from build123d import *

# Parameters (mm, degrees)
SKETCH021_R     = 10.25
PAD007_DEPTH    = 20
PAD007_FACE1_W  = 40
PAD007_FACE1_H  = 46.7452916506
PAD008_DEPTH    = 4
SKETCH022_R     = 1.75
POCKET007_DEPTH = 6.5
POCKET008_DEPTH = 4
SKETCH024_R     = 2.5
POCKET009_DEPTH = 29.501


with BuildPart() as part:
    # Sketch021 → Pad007 (new body, symmetric)
    with BuildSketch(Plane.XZ):
        with BuildLine():
            Line((23.3726458253, 0), (-23.3726458253, 0))
            Line((-23.3726458253, 0), (-26.8054242847, -7.3616171628))
            ThreePointArc((-26.8054242847, -7.3616171628), (-28, -12.75), (-26.8054242847, -18.1383828372))
            Line((-26.8054242847, -18.1383828372), (-23.3726458253, -25.5))
            Line((-23.3726458253, -25.5), (23.3726458253, -25.5))
            Line((23.3726458253, -25.5), (26.8054242847, -18.1383828372))
            ThreePointArc((26.8054242847, -18.1383828372), (28, -12.75), (26.8054242847, -7.3616171628))
            Line((23.3726458253, 0), (26.8054242847, -7.3616171628))
        make_face()
        with Locations((15.25, -12.75)):
            Circle(SKETCH021_R, mode=Mode.SUBTRACT)
        with Locations((-15.25, -12.75)):
            Circle(SKETCH021_R, mode=Mode.SUBTRACT)
        with BuildLine():
            Line((-7.6671245559, -2.5), (7.6671245559, -2.5))
            ThreePointArc((7.6671245559, -2.5), (2.5, -12.75), (7.6671245559, -23))
            Line((-7.6671245559, -23), (7.6671245559, -23))
            ThreePointArc((-7.6671245559, -23), (-2.5, -12.75), (-7.6671245559, -2.5))
        make_face(mode=Mode.SUBTRACT)
    extrude(amount=PAD007_DEPTH, both=True)

    # Pad007 Face1 → Pad008 (add)
    with BuildSketch(Plane(origin=(0, 0, 0), x_dir=(0, 1, 0), z_dir=(0, 0, 1))):
        Rectangle(PAD007_FACE1_W, PAD007_FACE1_H)
    extrude(amount=PAD008_DEPTH)

    # Sketch022 → Pocket007 (cut)
    with BuildSketch(Plane(origin=(0, 0, 4), x_dir=(-1, 0, 0), z_dir=(0, 0, 1))):
        with Locations((0, 10)):
            Circle(SKETCH022_R)
        with Locations((0, -10)):
            Circle(SKETCH022_R)
    extrude(amount=-POCKET007_DEPTH, mode=Mode.SUBTRACT)

    # Sketch023 (on Face6 of Pocket007) → Pocket008 (cut)
    with BuildSketch(Plane(origin=(0, 0, 4), x_dir=(-1, 0, 0), z_dir=(0, 0, 1))):
        Polygon((2.225, -3.8538130468), (4.45, 0), (2.225, 3.8538130468), (-2.225, 3.8538130468), (-4.45, 0), (-2.225, -3.8538130468), align=None)
    extrude(amount=-POCKET008_DEPTH, mode=Mode.SUBTRACT)

    # Sketch024 (on Face6 of Pocket008) → Pocket009 (cut, through all)
    with BuildSketch(Plane(origin=(0, 0, 4), x_dir=(-1, 0, 0), z_dir=(0, 0, 1))):
        Circle(SKETCH024_R)
    extrude(amount=-POCKET009_DEPTH, mode=Mode.SUBTRACT)


solid = part.part
Input: part model. Units: mm. Frame: model coordinates. A direction names the side the tool comes from. Give positions to 0.01 mm unless a question says otherwise; leave off trailing zeros. Loops run counter-clockwise (first coordinate to the right, second up) from the corner with the lowest first, then second, coordinate; pieces in that order, holes last. Notation, with made-up numbers: (-15.75, 20.5) -> (20.25, 20.5) arc R30 cw to (20.25, 45.5) -> close; hole circle Ø4 at (13.5, 16). An arc over 180 degrees is marked (long way). Answer as a JSON object with one key per item and string values. Group by question number.
Item 1: Pull-direction query (Z, two-part tool) for faces 4 (the flat face through (25.065, -0.28, -3.629)), 5 (the flat face through (-3.322, 1.954, 2.028)), 6 (the cylindrical face through (-2.5, -0.3, -12.9)), 7 (the flat face through (-4, 0, -2.5)); classes: released by +Z, released by -Z, zero draft, split by the parting line, or undercut.
Item 2: Reachability of faces 1 (the cylindrical face through (28, -0.3, -12.8)), 2 (the flat face through (23.373, 0, 2)), 3 (the flat face through (3.353, 1.9, 2.028)) from +Z, -Z, +X, -X, +Y, -Y: full face, straight path, thin tool, end or side. Return the list, or none.
Item 3: Line query: probe 1 along Y at (x, z) = (0, 0.75); probe 2 along Y at (x, z) = (0, -24.45); probe 3 along X at (y, z) = (4, -9.25). Output: solid intervals per line, ascending.
Item 4: Cut plane D-D, the plane z = 2.25. Return the cut outline in (x, y) (3 decimals), and give its area (3 significant figures).
Item 5: Pin query (flat end, axial travel): P1, Ø12, axis at y = -1, z = -22, coming from the +X side; P2, Ø1.2, axis at y = -7.5, z = 1.5, coming from the -X side; P3, Ø4, axis at y = -11, z = -20, coming from the +X side. Return the tip coordinate at first contact, or that it passes through.
Item 6: Cut plane C-C, the plane y = -10. Return the cut outline in (x, z).
Item 7: Cut plane A-A, the plane z = -12.75. Return the cut outline in (x, y).
Item 8: Cut plane B-B, the plane x = 0. Return the cut outline in (y, z), and give its area (3 significant figures).
Checks:
{
 "1": {"face 4": "released by +Z", "face 5": "zero draft", "face 6": "undercut", "face 7": "undercut"},
 "2": {"face 1": "+X, +Y, -Y", "face 2": "+Z, +X, +Y, -Y", "face 3": "+Z"},
 "3": {"probe 1": "y = -20 to -11.75, -8.25 to -3.85, 3.85 to 8.25, 11.75 to 20", "probe 2": "y = -20 to -2.5, 2.5 to 20", "probe 3": "x = -27.51 to -24.88, -5.62 to -2.99, 2.99 to 5.62, 24.88 to 27.51"},
 "4": {"outline": "(-23.373, -20) -> (23.373, -20) -> (23.373, 20) -> (-23.373, 20) -> close; hole (-4.45, 0) -> (-2.225, -3.854) -> (2.225, -3.854) -> (4.45, 0) -> (2.225, 3.854) -> (-2.225, 3.854) -> close; hole circle Ø3.5 at (0, -10); hole circle Ø3.5 at (0, 10)", "area": "1,800 mm²"},
 "5": {"P1": "stops at x = 27.58", "P2": "stops at x = -23.37", "P3": "stops at x = 26.87"},
 "6": {"outline": "(-26.81, -18.14) -> (-23.37, -25.5) -> (23.37, -25.5) -> (26.81, -18.14) arc R12.75 ccw to (26.81, -7.36) -> (23.37, 0) -> (23.37, 4) -> (1.75, 4) -> (1.75, -2.5) -> (7.67, -2.5) arc R12.75 ccw to (7.67, -23) -> (-7.67, -23) arc R12.75 ccw to (-7.67, -2.5) -> (-1.75, -2.5) -> (-1.75, 4) -> (-23.37, 4) -> (-23.37, 0) -> (-26.81, -7.36) arc R12.75 ccw to start; hole circle Ø20.5 at (-15.25, -12.75); hole circle Ø20.5 at (15.25, -12.75)"},
 "7": {"outline": "(-28, -20) -> (-25.5, -20) -> (-25.5, 20) -> (-28, 20) -> close; (-5, -20) -> (-2.5, -20) -> (-2.5, 20) -> (-5, 20) -> close; (2.5, -20) -> (5, -20) -> (5, 20) -> (2.5, 20) -> close; (25.5, -20) -> (28, -20) -> (28, 20) -> (25.5, 20) -> close"},
 "8": {"outline": "(-20, -25.5) -> (-2.5, -25.5) -> (-2.5, -23) -> (-20, -23) -> close; (-20, -2.5) -> (-11.75, -2.5) -> (-11.75, 4) -> (-20, 4) -> close; (-8.25, -2.5) -> (-2.5, -2.5) -> (-2.5, 0) -> (-3.85, 0) -> (-3.85, 4) -> (-8.25, 4) -> close; (2.5, -25.5) -> (20, -25.5) -> (20, -23) -> (2.5, -23) -> close; (2.5, -2.5) -> (8.25, -2.5) -> (8.25, 4) -> (3.85, 4) -> (3.85, 0) -> (2.5, 0) -> close; (11.75, -2.5) -> (20, -2.5) -> (20, 4) -> (11.75, 4) -> close", "area": "259 mm²"}
}
